from build123d import *

# Parameters (mm, degrees)
SKETCH1_R           = 1.2
BOSS_EXTRUDE1_DEPTH = 1.4
SKETCH2_W           = 7
SKETCH2_H           = 6.7
BOSS_EXTRUDE2_DEPTH = 8.8
SKETCH3_W           = 10
SKETCH3_H           = 7.6
BOSS_EXTRUDE3_DEPTH = 8.5
SKETCH4_R           = 4.05
BOSS_EXTRUDE4_DEPTH = 12.9


with BuildPart() as part:
    # Sketch1 → Boss-Extrude1 (new body)
    with BuildSketch(Plane(origin=(0, 0, 0), x_dir=(1, 0, 0), z_dir=(0, 1, 0))):
        with BuildLine():
            Line((-30.1, -12.675), (30.1, -12.675))
            ThreePointArc((30.1, -12.675), (30.807106781, -12.382106781), (31.1, -11.675))
            Line((31.1, -11.675), (31.1, 11.675))
            ThreePointArc((31.1, 11.675), (30.807106781, 12.382106781), (30.1, 12.675))
            Line((30.1, 12.675), (-30.1, 12.675))
            ThreePointArc((-30.1, 12.675), (-30.807106781, 12.382106781), (-31.1, 11.675))
            Line((-31.1, 11.675), (-31.1, -11.675))
            ThreePointArc((-31.1, -11.675), (-30.807106781, -12.382106781), (-30.1, -12.675))
        make_face()
        with Locations(Location((-27.9, 9.45, 0), (0, 0, 270))):
            Circle(SKETCH1_R, mode=Mode.SUBTRACT)
        with Locations(Location((-27.9, -9.45, 0), (0, 0, 270))):
            Circle(SKETCH1_R, mode=Mode.SUBTRACT)
        with Locations(Location((27.9, -9.45, 0), (0, 0, 270))):
            Circle(SKETCH1_R, mode=Mode.SUBTRACT)
        with Locations(Location((27.9, 9.45, 0), (0, 0, 270))):
            Circle(SKETCH1_R, mode=Mode.SUBTRACT)
    extrude(amount=BOSS_EXTRUDE1_DEPTH)

    # Sketch2 → Boss-Extrude2 (add)
    with BuildSketch(Plane(origin=(0, 1.4, 0), x_dir=(1, 0, 0), z_dir=(0, 1, 0))):
        with Locations((0, 8.825)):
            Rectangle(SKETCH2_W, SKETCH2_H)
    extrude(amount=BOSS_EXTRUDE2_DEPTH)

    # Sketch3 → Boss-Extrude3 (add)
    with BuildSketch(Plane(origin=(0, 1.4, 0), x_dir=(1, 0, 0), z_dir=(0, 1, 0))):
        with Locations((-20.4, -8.775)):
            Rectangle(SKETCH3_W, SKETCH3_H)
        with Locations((-7.56, -8.775)):
            Rectangle(SKETCH3_W, SKETCH3_H)
    boss_extrude3 = extrude(amount=BOSS_EXTRUDE3_DEPTH)

    # Mirror1: Boss-Extrude3 across plane
    add(boss_extrude3.mirror(Plane(origin=(0, 0, 0), x_dir=(0, 0, 1), z_dir=(1, 0, 0))))

    # Sketch4 → Boss-Extrude4 (add)
    with BuildSketch(Plane(origin=(0, 1.4, 0), x_dir=(1, 0, 0), z_dir=(0, 1, 0))):
        with Locations(Location((-18.7, 8.525, 0), (0, 0, 90))):
            Circle(SKETCH4_R)
    extrude(amount=BOSS_EXTRUDE4_DEPTH)


solid = part.part
Geometry check sheet. Reference: the model listing, model coordinates, mm. A direction names the side the tool comes from. Round coordinates to 2 decimals unless told otherwise and drop trailing zeros. Order: outer loops, then holes, each group sorted by start corner. A loop starts at its lowest first (then second) coordinate and runs counter-clockwise, first axis right, second up. Notation, with made-up numbers: M 81,12.5 L 99,12.5 A31 cw 99,48.5 Z; hole C 83.5,38.25 d5. An arc over 180 degrees is marked long. Write each question's results on one line, items separated by ' | '. Start each with the question number.
1. Set-up check for faces 1 (the face through (-3.5, 6, -9)), 2 (the face through (0, 6, -5.475)), 3 (the face through (-8, 6, 12.575)): record each of +Z, -Z, +X, -X, +Y, -Y from which the full face is reachable in a straight line by a thin tool's end or side.
2. Cross-section at D-D on x = -18.7. Record the boundary of the cut face in (y, z) (3 decimals), plus the area to 3 significant figures.
3. Material ranges on L1, parallel to X at y = 0.35, z = 9.45; L2, parallel to X at y = 7, z = 9.5; L3, parallel to Y at x = 2, z = -7.25, recorded low to high. Write a range as from..to.
4. Cross-section at A-A on x = 27.9. Record the boundary of the cut face in (y, z) (3 decimals).
5. Cross-section at B-B on y = 3. Record the boundary of the cut face in (x, z) (3 decimals), plus the area to 3 significant figures.
6. Draft check along Z on faces 4 (the face through (-26.71, 0.69, -9.61)), 5 (the face through (20, 6, 12.575)), 6 (the face through (-17.149, 7.76, -12.266)), 7 (the face through (20, 9.9, 9)). Enter one of: pulls with the +Z half, pulls with the -Z half, needs draft (parallel to the pull), parting line crosses it, or undercut.
7. Cross-section at C-C on z = 9.25. Record the boundary of the cut face in (x, y), plus the area to 3 significant figures.
8. Go/stop test with flat-tipped pins: P1, Ø10, axis at x = 10.5, z = -2, coming from the +Y side; P2, Ø7, axis at x = 10, y = 6.5, coming from the +Z side (3 decimals); P3, Ø2.5, axis at y = 7, z = 10, coming from the -X side; P4, Ø1.4, axis at x = 27.9, z = -9.45, coming from the +Y side. Record where each tip stops, or that it passes through.
Resolved:
1) face 1: -Z, +Y | face 2: +X, +Y | face 3: +Z, +X, -X, +Y
2) outline: M 0,-12.675 L 1.4,-12.675 L 1.4,-12.575 L 14.3,-12.575 L 14.3,-4.475 L 1.4,-4.475 L 1.4,4.975 L 9.9,4.975 L 9.9,12.575 L 1.4,12.575 L 1.4,12.675 L 0,12.675 Z | area: 205 mm2
3) L1: -31.1..-29.1, -26.7..26.7, 29.1..31.1 | L2: -25.4..-15.4, -12.56..-2.56, 2.56..12.56, 15.4..25.4 | L3: 0..10.2
4) outline: M 0,-12.675 L 1.4,-12.675 L 1.4,-10.65 L 0,-10.65 Z; M 0,-8.25 L 1.4,-8.25 L 1.4,8.25 L 0,8.25 Z; M 0,10.65 L 1.4,10.65 L 1.4,12.675 L 0,12.675 Z
5) outline: M -25.4,4.975 L -15.4,4.975 L -15.4,12.575 L -25.4,12.575 Z; C -18.7,-8.525 d8.1; M -12.56,4.975 L -2.56,4.975 L -2.56,12.575 L -12.56,12.575 Z; M -3.5,-12.175 L 3.5,-12.175 L 3.5,-5.475 L -3.5,-5.475 Z; M 2.56,4.975 L 12.56,4.975 L 12.56,12.575 L 2.56,12.575 Z; M 15.4,4.975 L 25.4,4.975 L 25.4,12.575 L 15.4,12.575 Z | area: 402 mm2
6) face 4: undercut | face 5: pulls with the +Z half | face 6: undercut | face 7: needs draft
7) outline: M -31.1,0 L -29.08,0 L -29.08,1.4 L -31.1,1.4 Z; M -26.72,0 L 26.72,0 L 26.72,1.4 L 25.4,1.4 L 25.4,9.9 L 15.4,9.9 L 15.4,1.4 L 12.56,1.4 L 12.56,9.9 L 2.56,9.9 L 2.56,1.4 L -2.56,1.4 L -2.56,9.9 L -12.56,9.9 L -12.56,1.4 L -15.4,1.4 L -15.4,9.9 L -25.4,9.9 L -25.4,1.4 L -26.72,1.4 Z; M 29.08,0 L 31.1,0 L 31.1,1.4 L 29.08,1.4 Z | area: 420 mm2
8) P1: y = 1.4 | P2: z = 12.575 | P3: x = -25.4 | P4: through
